Can you work these out from the model? Positions are in its coordinate system, mm. Give positions to 0.01 mm unless a question says otherwise; leave off trailing zeros. Loops run counter-clockwise (first coordinate to the right, second up) from the corner with the lowest first, then second, coordinate; pieces in that order, holes last. Notation, with made-up numbers: (-10, 63.25) - (44, 63.25) arc R21 ccw to (44, 74.25) - close; hole circle Ø2 at (43.25, 83). An arc over 180 degrees is marked (long way). Answer as a JSON object with one key per item and string values. Group by question number.
Item 1: Please list where these lines run through material, in increasing order: L1, parallel to Z at x = -15.5, y = -1; L2, parallel to Z at x = -22, y = -0.25; L3, parallel to X at y = -2.6, z = 43.5.
Item 2: Suppose I cut it at A-A on z = 68. Write out the boundary of the cut face in (x, y) (3 decimals), and give its area (3 significant figures).
Item 3: Suppose I cut it at C-C on y = -1.05. Count the separate pieces of the cut face and the enclosed holes in it, and give its area (3 significant figures).
Item 4: Thinking about a two-plate mould opening in X: for faces 1 (the cylindrical face through (113.09, -1.57, -104.83)), 2 (the flat face through (-2, 0, -71)), which applies, pulls with the +X half, pulls with the -X half, needs draft (parallel to the pull), parting line crosses it, or undercut?
Item 5: Suppose I cut it at B-B on x = -87. Write out the boundary of the cut face in (y, z) (3 decimals).
Item 6: Will this pin go through, and if not, where does the flat tip stop? pin 1 (2 mm diameter, centred on x = -18, z = -63.5, fed in from +Y).
from build123d import *

# Parameters (mm, degrees)
F0_W     = 330.2
F0_H     = 330.2
F3_DEPTH = 3.175
F4_DEPTH = 25.4


with BuildPart() as f3:
    # F0 (on Front) → F3 (new body)
    with BuildSketch(Plane.XZ):
        Rectangle(F0_W, F0_H)
    extrude(amount=F3_DEPTH)

    # F1 (on face) + F2 (on face) → F4 (cut)
    with BuildSketch(Plane.XZ):
        with BuildLine():
            ThreePointArc((-114.3, -33.3375), (-112.905096, -36.705096), (-109.5375, -38.1))
            Line((-109.5375, -38.1), (109.5375, -38.1))
            ThreePointArc((109.5375, -38.1), (112.905096, -36.705096), (114.3, -33.3375))
            Line((114.3, -33.3375), (114.3, 109.5375))
            ThreePointArc((114.3, 109.5375), (112.905096, 112.905096), (109.5375, 114.3))
            Line((109.5375, 114.3), (-109.5375, 114.3))
            ThreePointArc((-109.5375, 114.3), (-112.905096, 112.905096), (-114.3, 109.5375))
            Line((-114.3, 109.5375), (-114.3, -33.3375))
        make_face()
    with BuildSketch(Plane.XZ):
        with BuildLine():
            ThreePointArc((82.55, -98.754585), (98.425, -114.629585), (114.3, -98.754585))
            ThreePointArc((114.3, -98.754585), (98.425, -82.879585), (82.55, -98.754585))
        make_face()
        with BuildLine():
            ThreePointArc((-19.05, -98.754585), (-15.875, -101.929585), (-12.7, -98.754585))
            Line((-12.7, -98.754585), (-19.05, -98.754585))
        make_face()
        with BuildLine():
            Line((-19.05, -98.754585), (-12.7, -98.754585))
            ThreePointArc((-12.7, -98.754585), (-15.875, -95.579585), (-19.05, -98.754585))
        make_face()
        with BuildLine():
            Line((-50.8, -98.754585), (-44.45, -98.754585))
            ThreePointArc((-44.45, -98.754585), (-47.625, -95.579585), (-50.8, -98.754585))
        make_face()
        with BuildLine():
            ThreePointArc((-50.8, -98.754585), (-47.625, -101.929585), (-44.45, -98.754585))
            Line((-44.45, -98.754585), (-50.8, -98.754585))
        make_face()
        with BuildLine():
            Line((-82.55, -98.754585), (-76.2, -98.754585))
            ThreePointArc((-76.2, -98.754585), (-79.375, -95.579585), (-82.55, -98.754585))
        make_face()
        with BuildLine():
            ThreePointArc((-82.55, -98.754585), (-79.375, -101.929585), (-76.2, -98.754585))
            Line((-76.2, -98.754585), (-82.55, -98.754585))
        make_face()
        with BuildLine():
            ThreePointArc((-114.3, -98.754585), (-111.125, -101.929585), (-107.95, -98.754585))
            Line((-107.95, -98.754585), (-114.3, -98.754585))
        make_face()
        with BuildLine():
            Line((-114.3, -98.754585), (-107.95, -98.754585))
            ThreePointArc((-107.95, -98.754585), (-111.125, -95.579585), (-114.3, -98.754585))
        make_face()
    extrude(amount=F4_DEPTH, mode=Mode.SUBTRACT)


solid = f3.part
Worked out:
{
 "1": {"L1": "z = -165.1 to -101.91, -95.6 to -38.1, 114.3 to 165.1", "L2": "z = -165.1 to -38.1, 114.3 to 165.1", "L3": "x = -165.1 to -114.3, 114.3 to 165.1"},
 "2": {"outline": "(-165.1, -3.175) - (-114.3, -3.175) - (-114.3, 0) - (-165.1, 0) - close; (114.3, -3.175) - (165.1, -3.175) - (165.1, 0) - (114.3, 0) - close", "area": "323 mm2"},
 "3": {"separate pieces": "1", "enclosed holes": "6", "area": "73,300 mm2"},
 "4": {"face 1": "undercut", "face 2": "needs draft"},
 "5": {"outline": "(-3.175, -165.1) - (0, -165.1) - (0, -38.1) - (-3.175, -38.1) - close; (-3.175, 114.3) - (0, 114.3) - (0, 165.1) - (-3.175, 165.1) - close"},
 "6": {"pin 1": "stops at y = 0"}
}
